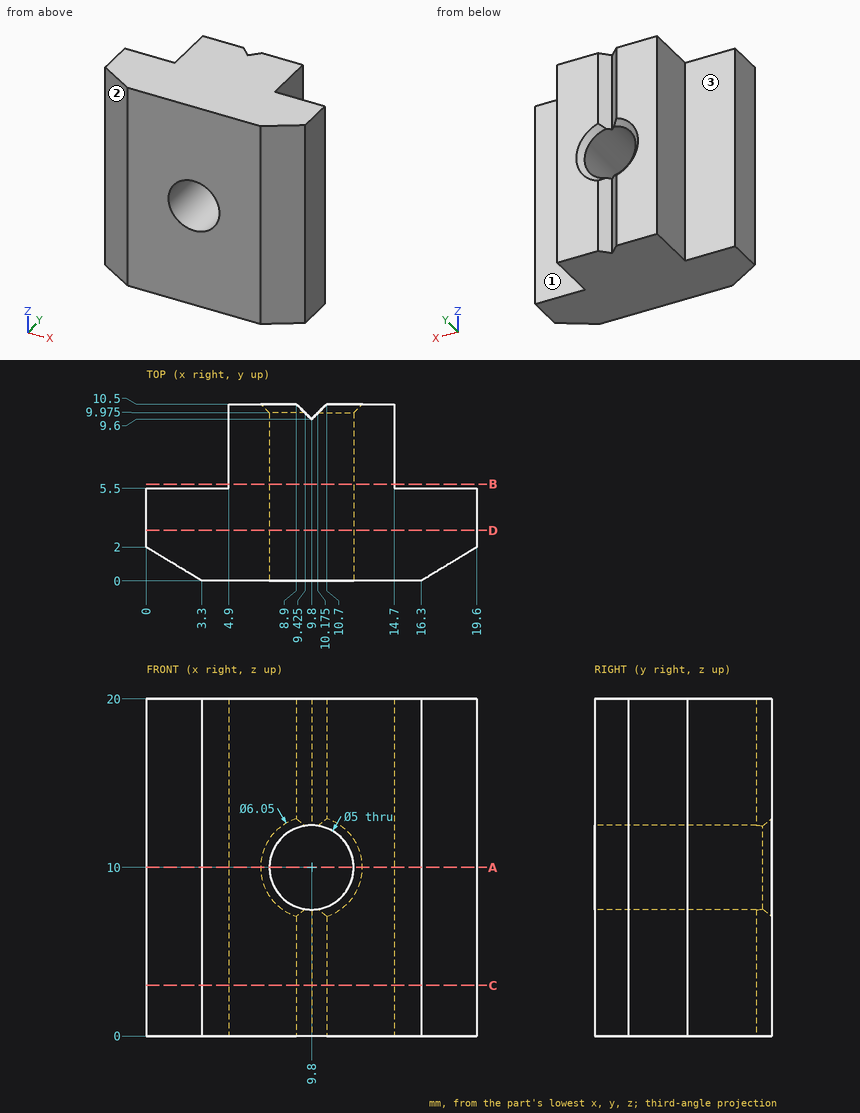
For this review, use the dimensioned drawing (mm, ordinates from the lowest corner) and the shaded views. A direction names the side the tool comes from. Round coordinates to 2 decimals unless told otherwise and drop trailing zeros. Write each loop counter-clockwise with the first axis right and the second up, starting at its lowest first coordinate (ties: lowest second). Pieces come first, ordered by that corner, then holes. Notation, with made-up numbers: (-34.75, 13.25) -> (-26.75, 13.25) arc R20 ccw to (-26.75, 26.25) -> close; hole circle Ø9 at (43.5, 10.25). An arc over 180 degrees is marked (long way). Use CSV: the item, a comma, the result in double quotes.
(1) Consider section B-B, the plane y = 5.75. Give the boundary of the cut face in (x, z).
Computed values:
outline,"(4.9, 0) -> (14.7, 0) -> (14.7, 20) -> (4.9, 20) -> close; hole circle Ø5 at (9.8, 10)"
(2) Consider section D-D, the plane y = 3. Give the boundary of the cut face in (x, z), plus the area to 3 significant figures.
Computed values:
outline,"(0, 0) -> (19.6, 0) -> (19.6, 20) -> (0, 20) -> close; hole circle Ø5 at (9.8, 10)"
area,"372 mm²"
(3) For the marked faces 1, 2 and 3, list the 3-axis set-ups (+Z, -Z, +X, -X, +Y, -Y) from which the entire face can be reached by the end or side of a thin tool; tool diameter is ignored.
Computed values:
face 1,"+Z, -Z, +X, +Y"
face 2,"+Z, -Z, -X, -Y"
face 3,"+Z, -Z, -X, +Y"
(4) Clearance check with flat-ended pins moving along their axes: P1, Ø2.5, axis at x = 3.5, z = 6.5, coming from the +Y side; P2, Ø3, axis at y = 8, z = 4.5, coming from the +X side; P3, Ø1.5, axis at y = 7, z = 6.5, coming from the -X side. State where each tip first meets the part, or that it passes through.
Computed values:
P1,"y = 5.5"
P2,"x = 14.7"
P3,"x = 4.9"
(5) To check wall thickness, follow L1, parallel to X at y = 5.75, z = 10; L2, parallel to X at y = 3.25, z = 10; L3, parallel to Z at x = 9.8, y = 2.75. State the ranges of each line that lie inside material, in increasing order. Write a range as [from, to].
Computed values:
L1,"[4.9, 7.3], [12.3, 14.7]"
L2,"[0, 7.3], [12.3, 19.6]"
L3,"[0, 7.5], [12.5, 20]"
(6) Consider section C-C, the plane z = 3. Give the boundary of the cut face in (x, y).
Computed values:
outline,"(0, 2) -> (3.3, 0) -> (16.3, 0) -> (19.6, 2) -> (19.6, 5.5) -> (14.7, 5.5) -> (14.7, 10.5) -> (10.7, 10.5) -> (9.8, 9.6) -> (8.9, 10.5) -> (4.9, 10.5) -> (4.9, 5.5) -> (0, 5.5) -> close"
(7) Consider section A-A, the plane z = 10. Give the boundary of the cut face in (x, y) (3 decimals), plus the area to 3 significant figures.
Computed values:
outline,"(0, 2) -> (3.3, 0) -> (7.3, 0) -> (7.3, 9.975) -> (6.775, 10.5) -> (4.9, 10.5) -> (4.9, 5.5) -> (0, 5.5) -> close; (12.3, 0) -> (16.3, 0) -> (19.6, 2) -> (19.6, 5.5) -> (14.7, 5.5) -> (14.7, 10.5) -> (12.825, 10.5) -> (12.3, 9.975) -> close"
area,"97.4 mm²"
